For this review, use the dimensioned drawing (mm, ordinates from the lowest corner) and the shaded views. A direction names the side the tool comes from. Give positions to 0.01 mm unless a question says otherwise; leave off trailing zeros. Order: outer loops, then holes, each group sorted by start corner. A loop starts at its lowest first (then second) coordinate and runs counter-clockwise, first axis right, second up. Notation, with made-up numbers: (-19, 8) -> (10, 8) arc R29 ccw to (10, 29) -> close; hole circle Ø4 at (-27, 65). An arc over 180 degrees is marked (long way). Answer as a JSON object with one key per item and string values. Group by question number.
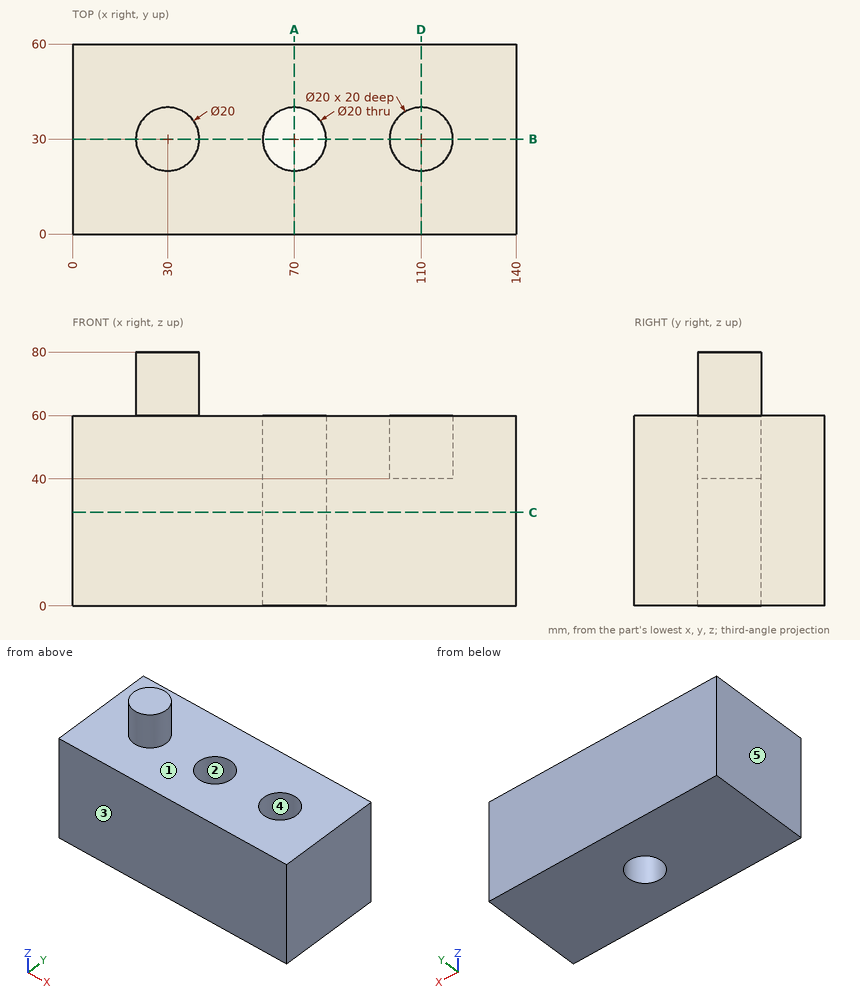
1. Machinability: for the marked faces 4 and 5, which of the approach directions +Z, -Z, +X, -X, +Y, -Y give a long, thin tool a straight path to every point of the face, cutting with its end or side? Answer none if there is none.
2. Draft analysis for pull direction Y (two halves, no side actions). For the marked faces 1, 2 and 3, state which applies: pulls with the +Y half, pulls with the -Y half, needs draft (parallel to the pull), parting line crosses it, or undercut.
3. For pin 1 (4 mm diameter, centred on x = 67, y = 19, fed in from +Z), flat-tipped, find the tip position at first contact; note if it passes through.
4. Take a section at A-A on x = 70. Give the boundary of the cut face in (y, z).
5. Take a section at D-D on x = 110. Give the boundary of the cut face in (y, z).
6. Take a section at C-C on z = 29.5. Give the boundary of the cut face in (x, y).
7. Take a section at B-B on y = 30. Give the boundary of the cut face in (x, z), plus the area to 3 significant figures.
8. For probe 1 along Y at (x, z) = (110, 49.75); probe 2 along X at (y, z) = (28, 49); probe 3 along X at (y, z) = (32.5, 42.5), list the stretches that pass through material, from the lowest coordinate up. Write a range as [from, to].
Checks:
{
 "1": {"face 4": "+Z", "face 5": "+Z, -Z, -X, +Y, -Y"},
 "2": {"face 1": "needs draft", "face 2": "undercut", "face 3": "pulls with the -Y half"},
 "3": {"pin 1": "stops at z = 60"},
 "4": {"outline": "(0, 0) -> (20, 0) -> (20, 60) -> (0, 60) -> close; (40, 0) -> (60, 0) -> (60, 60) -> (40, 60) -> close"},
 "5": {"outline": "(0, 0) -> (60, 0) -> (60, 60) -> (40, 60) -> (40, 40) -> (20, 40) -> (20, 60) -> (0, 60) -> close"},
 "6": {"outline": "(0, 0) -> (140, 0) -> (140, 60) -> (0, 60) -> close; hole circle Ø20 at (70, 30)"},
 "7": {"outline": "(0, 0) -> (60, 0) -> (60, 60) -> (40, 60) -> (40, 80) -> (20, 80) -> (20, 60) -> (0, 60) -> close; (80, 0) -> (140, 0) -> (140, 60) -> (120, 60) -> (120, 40) -> (100, 40) -> (100, 60) -> (80, 60) -> close", "area": "7,200 mm2"},
 "8": {"probe 1": "y = [0, 20], [40, 60]", "probe 2": "x = [0, 60.2], [79.8, 100.2], [119.8, 140]", "probe 3": "x = [0, 60.32], [79.68, 100.32], [119.68, 140]"}
}
